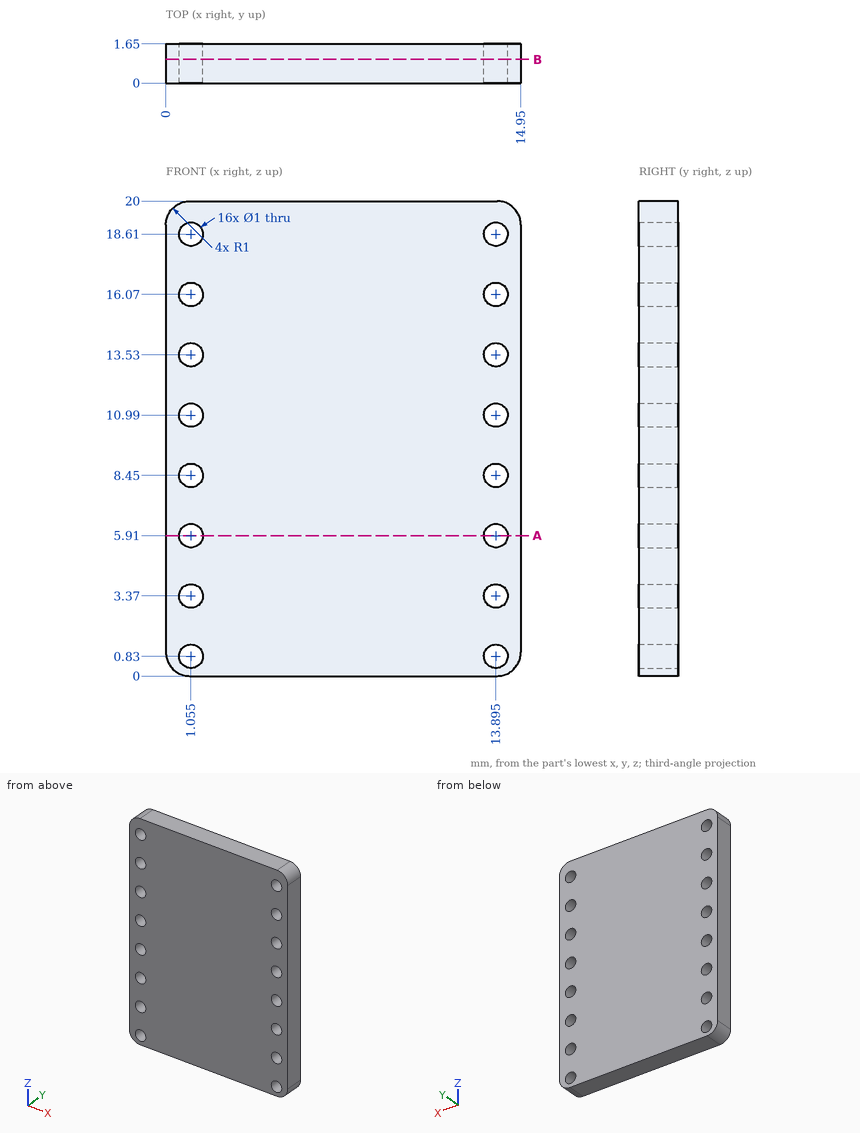
For this review, use the dimensioned drawing (mm, ordinates from the lowest corner) and the shaded views. Round coordinates to 2 decimals unless told otherwise and drop trailing zeros. Order: outer loops, then holes, each group sorted by start corner. A loop starts at its lowest first (then second) coordinate and runs counter-clockwise, first axis right, second up. Notation, with made-up numbers: M -6.5,4.25 L 2.5,4.25 A24 ccw 2.5,20.25 Z; hole C 20,-4.75 d9. An arc over 180 degrees is marked long. Use a Markdown table: item, result. Add a question column.
Item 1: Add section B-B, the plane y = 1. State how many separate pieces and enclosed holes the cut face has, then the cut area to 3 significant figures.
Item 2: To check wall thickness, follow line 1 along X through (y, z) = (1.05, 8.5); line 2 along X through (y, z) = (0.3, 16.25). State the ranges of each line that lie inside material, in increasing order.
Item 3: Add section A-A, the plane z = 5.91. Give the boundary of the cut face in (x, y) (3 decimals).
Geometry results:
| question | item | result |
|---|---|---|
| 1 | separate pieces | 1 |
| 1 | enclosed holes | 16 |
| 1 | area | 286 mm² |
| 2 | line 1 | x = 0 to 0.56, 1.55 to 13.4, 14.39 to 14.95 |
| 2 | line 2 | x = 0 to 0.59, 1.52 to 13.43, 14.36 to 14.95 |
| 3 | outline | M 0,0 L 0.555,0 L 0.555,1.65 L 0,1.65 Z; M 1.555,0 L 13.395,0 L 13.395,1.65 L 1.555,1.65 Z; M 14.395,0 L 14.95,0 L 14.95,1.65 L 14.395,1.65 Z |
